Model file for the job. Use its own axes, mm. Face numbers are marked on the shaded views. A direction names the side the tool comes from. Round coordinates to 2 decimals unless told otherwise and drop trailing zeros. Order: outer loops, then holes, each group sorted by start corner. A loop starts at its lowest first (then second) coordinate and runs counter-clockwise, first axis right, second up. Notation, with made-up numbers: (45.5, 72) -> (88.5, 72) arc R31 ccw to (88.5, 99) -> close; hole circle Ø3 at (-12, 20.5). An arc over 180 degrees is marked (long way). Use CSV: the item, a comma, the result in double quotes.
```python
from build123d import *

# Parameters (mm, degrees)
SKETCH1_R                   = 20.5
BOSS_EXTRUDE1_DEPTH         = 20
BOSS_EXTRUDE3_START         = -20
SKETCH6_R                   = 55
SKETCH6_R_2                 = 20.5
BOSS_EXTRUDE3_DEPTH         = 20
SKETCH2_R                   = 23.5
CUT_EXTRUDE1_DEPTH          = 16
SKETCH4_W                   = 85
SKETCH4_H                   = 8
BOSS_EXTRUDE2_DEPTH         = 3
SKETCH3_R                   = 3.25
CUT_EXTRUDE2_DEPTH          = 153.164384795
SKETCH5_R                   = 5.5
CUT_EXTRUDE3_DEPTH          = 4.5
FILLET1_R                   = 5
M8_TAPPED_HOLE1_D           = 6.8
M8_TAPPED_HOLE1_DEPTH       = 16
M8_TAPPED_HOLE1_CSINK_D     = 8.05
M8_TAPPED_HOLE1_CSINK_ANGLE = 90
M8_TAPPED_HOLE1_TIP         = 2.042926105


with BuildPart() as part:
    # Sketch1 → Boss-Extrude1 (new body)
    with BuildSketch(Plane.XY):
        with BuildLine():
            Line((0, 40), (-140, 40))
            Line((-140, 40), (-140, -40))
            Line((-140, -40), (0, -40))
            ThreePointArc((0, -40), (40, 0), (0, 40))
        make_face()
        Circle(SKETCH1_R, mode=Mode.SUBTRACT)
    extrude(amount=BOSS_EXTRUDE1_DEPTH)

    # Sketch6 → Boss-Extrude3 (add)
    with BuildSketch(Plane.XY.offset(20).offset(BOSS_EXTRUDE3_START)):
        Circle(SKETCH6_R)
        Circle(SKETCH6_R_2, mode=Mode.SUBTRACT)
    extrude(amount=BOSS_EXTRUDE3_DEPTH)

    # Sketch2 → Cut-Extrude1 (cut)
    with BuildSketch(Plane.XY.offset(20)):
        Circle(SKETCH2_R)
    extrude(amount=-CUT_EXTRUDE1_DEPTH, mode=Mode.SUBTRACT)

    # Sketch4 → Boss-Extrude2 (add)
    with BuildSketch(Plane(origin=(0, 0, 0), x_dir=(-1, 0, 0), z_dir=(0, 0, -1))):
        with Locations((97.5, -25)):
            Rectangle(SKETCH4_W, SKETCH4_H)
        with Locations((97.5, 15)):
            Rectangle(SKETCH4_W, SKETCH4_H)
    extrude(amount=BOSS_EXTRUDE2_DEPTH)

    # Sketch3 → Cut-Extrude2 (cut, through all)
    with BuildSketch(Plane.XY.offset(20)):
        with Locations((-63.6, 15)):
            Circle(SKETCH3_R)
        with Locations((-130, 15)):
            Circle(SKETCH3_R)
        with Locations((-130, -25)):
            Circle(SKETCH3_R)
        with Locations((-63.6, -25)):
            Circle(SKETCH3_R)
    extrude(amount=-CUT_EXTRUDE2_DEPTH, mode=Mode.SUBTRACT)

    # Sketch5 → Cut-Extrude3 (cut)
    with BuildSketch(Plane.XY.offset(20)):
        with Locations((-130, 15)):
            Circle(SKETCH5_R)
        with Locations((-63.6, 15)):
            Circle(SKETCH5_R)
        with Locations((-63.6, -25)):
            Circle(SKETCH5_R)
        with Locations((-130, -25)):
            Circle(SKETCH5_R)
    extrude(amount=-CUT_EXTRUDE3_DEPTH, mode=Mode.SUBTRACT)

    # Fillet1
    fillet1_edges = [part.edges().sort_by_distance(p)[0] for p in [
        (-140, -40, 10),
        (-140, 40, 10),
    ]]
    fillet(fillet1_edges, radius=FILLET1_R)

    # M8 Tapped Hole1
    with Locations(Plane.XY.offset(20)):
        with Locations((30.759144982, 30.759144982), (-30.759144982, 30.759144982), (-30.759144982, -30.759144982), (30.759144982, -30.759144982)):
            CounterSinkHole(M8_TAPPED_HOLE1_D / 2, M8_TAPPED_HOLE1_CSINK_D / 2, depth=M8_TAPPED_HOLE1_DEPTH, counter_sink_angle=M8_TAPPED_HOLE1_CSINK_ANGLE)
            with Locations((0, 0, -(M8_TAPPED_HOLE1_DEPTH + M8_TAPPED_HOLE1_TIP / 2))):  # 118° drill point
                Cone(0, M8_TAPPED_HOLE1_D / 2, M8_TAPPED_HOLE1_TIP, mode=Mode.SUBTRACT)


solid = part.part
```
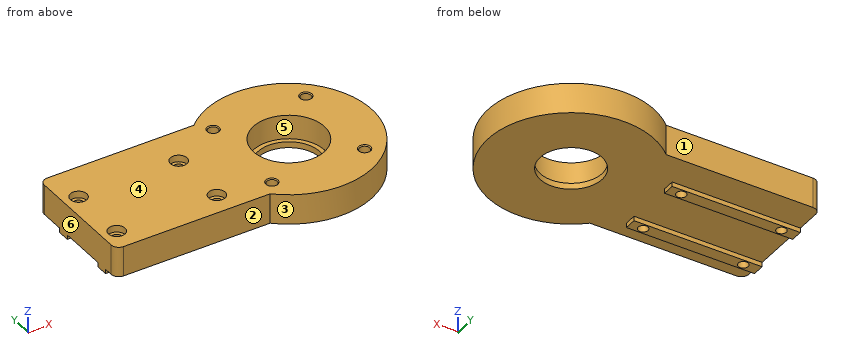
Q1. Probe line 1 along Y through (x, z) = (-130, 11.5); line 2 along Y through (x, z) = (-63.6, 16.9); line 3 along Y through (x, z) = (0.5, 15.25). List the from-to ranges inside material, lowest first.
From the geometry:
line 1,"y = -40 to -28.25, -21.75 to 11.75, 18.25 to 40"
line 2,"y = -40 to -30.5, -19.5 to 9.5, 20.5 to 40"
line 3,"y = -55 to -23.49, 23.49 to 55"
Q2. Mould opens along X. For the marked faces 3, 4, 5 and 6 say: +X half, -X half, draft (parallel to the pull), parting line (faces both ways), or undercut.
From the geometry:
face 3,"parting line"
face 4,"draft"
face 5,"undercut"
face 6,"-X half"
Q3. Cut at A-A (y = 0). Give the cut face in (x, z), plus the area to 3 significant figures.
From the geometry:
outline,"(-140, 0) -> (-20.5, 0) -> (-20.5, 4) -> (-23.5, 4) -> (-23.5, 20) -> (-140, 20) -> close; (20.5, 0) -> (55, 0) -> (55, 20) -> (23.5, 20) -> (23.5, 4) -> (20.5, 4) -> close"
area,"2,980 mm²"
Q4. Which spindle directions (+Z, -Z, +X, -X, +Y, -Y) get a long thin tool onto all of the face, cutting with end or side? Do the marked faces 1 and 2. Say none if no direction does.
From the geometry:
face 1,"+Z, -Z, -X, +Y"
face 2,"+Z, -Z, -X, -Y"
Q5. Cut at D-D (z = 6.5). State how many separate pieces and enclosed holes the cut face has, plus the area to 3 significant figures.
From the geometry:
separate pieces,"1"
enclosed holes,"9"
area,"14,700 mm²"
Q6. Cut at B-B (x = 0). Give the cut face in (y, z), plus the area to 3 significant figures.
From the geometry:
outline,"(-55, 0) -> (-20.5, 0) -> (-20.5, 4) -> (-23.5, 4) -> (-23.5, 20) -> (-55, 20) -> close; (20.5, 0) -> (55, 0) -> (55, 20) -> (23.5, 20) -> (23.5, 4) -> (20.5, 4) -> close"
area,"1,280 mm²"
Q7. Cut at C-C (x = -63.6). Give the cut face in (y, z), plus the area to 3 significant figures.
From the geometry:
outline,"(-40, 0) -> (-29, 0) -> (-29, -3) -> (-28.25, -3) -> (-28.25, 15.5) -> (-30.5, 15.5) -> (-30.5, 20) -> (-40, 20) -> close; (-21.75, -3) -> (-21, -3) -> (-21, 0) -> (11, 0) -> (11, -3) -> (11.75, -3) -> (11.75, 15.5) -> (9.5, 15.5) -> (9.5, 20) -> (-19.5, 20) -> (-19.5, 15.5) -> (-21.75, 15.5) -> close; (18.25, -3) -> (19, -3) -> (19, 0) -> (40, 0) -> (40, 20) -> (20.5, 20) -> (20.5, 15.5) -> (18.25, 15.5) -> close"
area,"1,310 mm²"
Q8. Pin check, flat tips, straight feed: pin 1 (9 mm diameter, centred on x = -130, y = -25, fed in from -Z); pin 2 (7.5 mm diameter, centred on x = -63.6, y = -25, fed in from +Z); pin 3 (8 mm diameter, centred on x = -64.5, z = 14.5, fed in from +Y); pin 4 (1.5 mm diameter, centred on y = 17, z = -1, fed in from +X). Stop position of each tip, or through.
From the geometry:
pin 1,"stops at z = -3"
pin 2,"stops at z = 15.5"
pin 3,"stops at y = 40"
pin 4,"stops at x = -55"
